Autodesk Inventor part; units mm, degrees
ref_plane "YZ Plane" through (0, 0, 0) normal (1, 0, 0) x (0, 1, 0)
ref_plane "XZ Plane" through (0, 0, 0) normal (0, 1, 0) x (-1, 0, 0)
ref_plane "XY Plane" through (0, 0, 0) normal (0, 0, 1) x (1, 0, 0)
sketch "Sketch1" plane through (0, 0, 0) normal (0, 0, 1) x (1, 0, 0)
  line L0 (-15.1032, 11.1381) -> (-28.4636, 11.1381)
  line L1 (-28.4636, 11.1381) -> (-28.4636, 26.8861)
  line L2 (-28.4636, 26.8861) -> (-15.1032, 26.8861)
  line L3 (-15.1032, 26.8861) -> (-15.1032, 11.1381)
  dimension "d0" = 13.3604
  dimension "d1" = 15.748
extrude "Extrusion1" add sketch "Sketch1" along normal blind 13.3096
sketch "Sketch2" plane through (0, 0, 13.3096) normal (0, 0, 1) x (1, 0, 0)
  line L0 (-28.4636, 11.1381) -> (-28.4636, 26.8861)
  line L1 (-15.1032, 11.1381) -> (-28.4636, 11.1381)
  line L2 (-15.1032, 26.8861) -> (-15.1032, 11.1381)
  line L3 (-28.4636, 26.8861) -> (-15.1032, 26.8861)
  line L4 (-23.79, 26.3273) -> (-19.7768, 26.3273)
  line L5 (-19.7768, 26.3273) -> (-19.7768, 24.0413)
  line L6 (-19.7768, 24.0413) -> (-23.79, 24.0413)
  line L7 (-23.79, 24.0413) -> (-23.79, 26.3273)
  line L8 (-25.06, 24.0413) -> (-18.5068, 24.0413)
  line L9 (-18.5068, 24.0413) -> (-18.5068, 22.8221)
  line L10 (-18.5068, 22.8221) -> (-25.06, 22.8221)
  line L11 (-25.06, 22.8221) -> (-25.06, 24.0413)
  line L12 (-16.5764, 22.8221) -> (-26.9904, 22.8221)
  line L13 (-26.9904, 22.8221) -> (-26.9904, 15.1259)
  line L14 (-26.9904, 15.1259) -> (-16.5764, 15.1259)
  line L15 (-16.5764, 15.1259) -> (-16.5764, 22.8221)
  line L16 (-25.06, 15.1259) -> (-18.5068, 15.1259)
  line L17 (-18.5068, 15.1259) -> (-18.5068, 14.0337)
  line L18 (-18.5068, 14.0337) -> (-25.06, 14.0337)
  line L19 (-25.06, 14.0337) -> (-25.06, 15.1259)
  dimension "d4" = 0.5588
  dimension "d5" = 4.6736
  dimension "d6" = 4.6736
  dimension "d7" = 2.286
  dimension "d9" = 1.27
  dimension "d10" = 1.27
  dimension "d11" = 1.2192
  dimension "d13" = 6.5532
  dimension "d14" = 1.9304
  dimension "d15" = 1.9304
  dimension "d16" = 10.414
  dimension "d17" = 7.6962
  dimension "d18" = 1.9304
  dimension "d19" = 1.9304
  dimension "d20" = 1.0922
  dimension "d21" = 2.8956
extrude "Extrusion2" cut sketch "Sketch2" against normal blind 14.1478 contours L4 L5 L6 L7 | L6 L8 L9 L10 L11 | L10 L12 L15 L14 L13 | L14 L17 L18 L19
sketch "Sketch3" plane through (0, 0, 0) normal (0, 0, -1) x (-1, 0, 0)
  line L0 (15.1032, 11.1381) -> (28.4636, 11.1381)
  line L1 (28.4636, 11.1381) -> (28.4636, 26.8861)
  line L2 (28.4636, 26.8861) -> (15.1032, 26.8861)
  line L3 (15.1032, 26.8861) -> (15.1032, 11.1381)
extrude "Extrusion3" add sketch "Sketch3" against normal blind 0.127
sketch "Sketch4" plane through (0, 0, 0.127) normal (0, 0, 1) x (1, 0, 0)
  line L0 (-25.06, 14.0337) -> (-25.06, 15.1259)
  line L1 (-18.5068, 14.0337) -> (-25.06, 14.0337)
  line L2 (-18.5068, 15.1259) -> (-18.5068, 14.0337)
  line L3 (-22.8629, 14.0337) -> (-22.6089, 14.0337)
  line L4 (-22.6089, 14.0337) -> (-22.6089, 16.4931)
  line L5 (-22.6089, 16.4931) -> (-22.8629, 16.4931)
  line L6 (-22.8629, 16.4931) -> (-22.8629, 14.0337)
  line L7 (-22.2279, 14.0337) -> (-21.9739, 14.0337)
  line L8 (-21.9739, 14.0337) -> (-21.9739, 16.4931)
  line L9 (-21.9739, 16.4931) -> (-22.2279, 16.4931)
  line L10 (-22.2279, 16.4931) -> (-22.2279, 14.0337)
  line L11 (-21.5929, 14.0337) -> (-21.3389, 14.0337)
  line L12 (-21.3389, 14.0337) -> (-21.3389, 16.4931)
  line L13 (-21.3389, 16.4931) -> (-21.5929, 16.4931)
  line L14 (-21.5929, 16.4931) -> (-21.5929, 14.0337)
  line L15 (-20.9579, 14.0337) -> (-20.7039, 14.0337)
  line L16 (-20.7039, 14.0337) -> (-20.7039, 16.4931)
  line L17 (-20.7039, 16.4931) -> (-20.9579, 16.4931)
  line L18 (-20.9579, 16.4931) -> (-20.9579, 14.0337)
  dimension "d26" = 0.254
  dimension "d27" = 0.254
  dimension "d28" = 0.254
  dimension "d29" = 0.254
  dimension "d30" = 0.381
  dimension "d31" = 0.381
  dimension "d32" = 0.381
  dimension "d33" = 2.1971
  dimension "d34" = 2.1971
extrude "Extrusion4" add sketch "Sketch4" along normal blind 6.4516
sketch "Sketch5" plane through (-22.8629, 14.0337, 0.127) normal (-1, 0, 0) x (0, 0, 1)
  line L0 (6.4516, 0) -> (6.4516, 2.4594)
  line L1 (0, 2.4594) -> (6.4516, 2.4594)
  line L2 (6.4516, 0) -> (0.1115, 2.4594)
extrude "Extrusion5" cut sketch "Sketch5" against normal blind 3.81
fillet "Fillet1" radius 0.127 8 edges at (-22.8629, 15.2634, 3.4085) (-22.6089, 15.2634, 3.4085) (-21.9739, 15.2634, 3.4085) (-22.2279, 15.2634, 3.4085) (-21.5929, 15.2634, 3.4085) (-21.3389, 15.2634, 3.4085) (-20.9579, 15.2634, 3.4085) (-20.7039, 15.2634, 3.4085)
sketch "Sketch6" plane through (0, 0, 0.127) normal (0, 0, 1) x (1, 0, 0)
  line L0 (-22.6089, 16.4001) -> (-22.6089, 14.0337)
  line L1 (-21.9739, 16.4001) -> (-21.9739, 14.0337)
  line L2 (-21.3389, 16.4001) -> (-21.3389, 14.0337)
  line L3 (-20.7039, 16.4001) -> (-20.7039, 14.0337)
  line L4 (-18.5068, 14.0337) -> (-20.7039, 14.0337)
  line L5 (-22.8629, 14.0337) -> (-25.06, 14.0337)
  line L6 (-22.8629, 14.0337) -> (-22.8629, 16.4001)
  line L7 (-25.0727, 14.0337) -> (-22.8629, 14.0337)
  line L8 (-22.8629, 14.0337) -> (-22.8629, 15.1259)
  line L9 (-22.8629, 15.1259) -> (-25.0727, 15.1259)
  line L10 (-25.0727, 15.1259) -> (-25.0727, 14.0337)
  line L11 (-22.6089, 15.1259) -> (-22.2279, 15.1259)
  line L12 (-22.2279, 15.1259) -> (-22.2279, 14.0337)
  line L13 (-22.2279, 14.0337) -> (-22.6089, 14.0337)
  line L14 (-22.6089, 14.0337) -> (-22.6089, 15.1259)
  line L15 (-21.9739, 15.1259) -> (-21.5929, 15.1259)
  line L16 (-21.5929, 15.1259) -> (-21.5929, 14.0337)
  line L17 (-21.5929, 14.0337) -> (-21.9739, 14.0337)
  line L18 (-21.9739, 14.0337) -> (-21.9739, 15.1259)
  line L19 (-21.3389, 15.1259) -> (-20.9579, 15.1259)
  line L20 (-20.9579, 15.1259) -> (-20.9579, 14.0337)
  line L21 (-20.9579, 14.0337) -> (-21.3389, 14.0337)
  line L22 (-21.3389, 14.0337) -> (-21.3389, 15.1259)
  line L23 (-20.7039, 15.1259) -> (-18.4941, 15.1259)
  line L24 (-18.4941, 15.1259) -> (-18.4941, 14.0337)
  line L25 (-18.4941, 14.0337) -> (-20.7039, 14.0337)
  line L26 (-20.7039, 14.0337) -> (-20.7039, 15.1259)
  line L27 (-22.8629, 14.0337) -> (-25.0727, 14.0337)
  line L28 (-25.0727, 14.0337) -> (-25.0727, 15.1259)
  line L29 (-25.0727, 15.1259) -> (-22.8629, 15.1259)
  line L30 (-22.8629, 15.1259) -> (-22.8629, 14.0337)
  line L31 (-20.7039, 15.1259) -> (-18.4941, 15.1259)
  line L32 (-18.4941, 15.1259) -> (-18.4941, 14.0337)
  line L33 (-18.4941, 14.0337) -> (-20.7039, 14.0337)
  line L34 (-20.7039, 14.0337) -> (-20.7039, 15.1259)
  point P0 (-25.06, 15.1259)
  dimension "d40" = 1.0922
  dimension "d41" = 1.0922
  dimension "d42" = 0
  dimension "d43" = 0
  dimension "d44" = 0
  dimension "d45" = 0
  dimension "d46" = 2.2098
  dimension "d47" = 2.2098
extrude "Extrusion6" add sketch "Sketch6" along normal blind 6.4516
sketch "Sketch7" plane through (0, 0, 0.127) normal (0, 0, 1) x (1, 0, 0)
  line L0 (-22.8629, 15.1259) -> (-22.6089, 15.1259)
  line L1 (-22.6089, 15.1259) -> (-22.6089, 22.5284)
  line L2 (-22.6089, 22.5284) -> (-22.8629, 22.5284)
  line L3 (-22.8629, 22.5284) -> (-22.8629, 15.1259)
  line L4 (-22.2279, 15.1259) -> (-21.9739, 15.1259)
  line L5 (-21.9739, 15.1259) -> (-21.9739, 22.5284)
  line L6 (-21.9739, 22.5284) -> (-22.2279, 22.5284)
  line L7 (-22.2279, 22.5284) -> (-22.2279, 15.1259)
  line L8 (-21.5929, 15.1259) -> (-21.3389, 15.1259)
  line L9 (-21.3389, 15.1259) -> (-21.3389, 22.5284)
  line L10 (-21.3389, 22.5284) -> (-21.5929, 22.5284)
  line L11 (-21.5929, 22.5284) -> (-21.5929, 15.1259)
  line L12 (-20.9579, 15.1259) -> (-20.7039, 15.1259)
  line L13 (-20.7039, 15.1259) -> (-20.7039, 22.5284)
  line L14 (-20.7039, 22.5284) -> (-20.9579, 22.5284)
  line L15 (-20.9579, 22.5284) -> (-20.9579, 15.1259)
  line L16 (-22.9407, 16.4931) -> (-20.3193, 16.4931)
  line L17 (-20.7381, 16.4931) -> (-20.9579, 16.4931)
  line L18 (-20.9579, 16.4931) -> (-20.9579, 22.5284)
  line L19 (-20.9579, 22.5284) -> (-20.7381, 22.5284)
  line L20 (-21.5929, 22.5284) -> (-21.3731, 22.5284)
  line L21 (-21.3731, 16.4931) -> (-21.5929, 16.4931)
  line L22 (-21.5929, 16.4931) -> (-21.5929, 22.5284)
  line L23 (-20.7039, 16.4931) -> (-20.9579, 16.4931)
  line L24 (-20.9579, 16.4931) -> (-20.9579, 22.5284)
  line L25 (-20.9579, 22.5284) -> (-20.7039, 22.5284)
  line L26 (-20.7039, 22.5284) -> (-20.7039, 16.4931)
  line L27 (-21.5929, 22.5284) -> (-21.3389, 22.5284)
  line L28 (-21.3389, 22.5284) -> (-21.3389, 16.4931)
  line L29 (-21.3389, 16.4931) -> (-21.5929, 16.4931)
  line L30 (-21.5929, 16.4931) -> (-21.5929, 22.5284)
  line L31 (-21.9739, 16.4931) -> (-22.2279, 16.4931)
  line L32 (-22.2279, 16.4931) -> (-22.2279, 22.5284)
  line L33 (-22.2279, 22.5284) -> (-21.9739, 22.5284)
  line L34 (-21.9739, 22.5284) -> (-21.9739, 16.4931)
  line L35 (-22.8629, 22.5284) -> (-22.6089, 22.5284)
  line L36 (-22.6089, 22.5284) -> (-22.6089, 16.4931)
  line L37 (-22.6089, 16.4931) -> (-22.8629, 16.4931)
  line L38 (-22.8629, 16.4931) -> (-22.8629, 22.5284)
extrude "Extrusion7" cut sketch "Sketch7" against normal blind 127 contours L15 L14 L13 L16 | L11 L10 L9 L16 | L7 L6 L5 L16 | L3 L2 L1 L16
equation "\"d6\" = d5"
equation "\"d10\" = d9"
equation "\"d15\" = d14"
equation "\"d27\" = d26"
equation "\"d28\" = d27"
equation "\"d29\" = d28"
equation "\"d31\" = d30"
equation "\"d32\" = d31"
equation "\"d40\" = d41"
equation "\"d47\" = d46"
properties part number "2009_CTS_EatherNetPort"
Geometry: final body of the model. Coordinates: model frame, mm. Coordinates: 2 decimals unless noted, no trailing zeros. Order: outer loops, then holes, each group sorted by start corner. A loop starts at its lowest first (then second) coordinate and runs counter-clockwise, first axis right, second up. Notation, with made-up numbers: M 43,75 L 83,75 A26 cw 83,97 Z; hole C 73.25,-4 d2. An arc over 180 degrees is marked long. Answer in a Markdown table with one row per item. Add a question column.
Q1. Line query: L1, parallel to X at y = 21, z = 7.25; L2, parallel to Y at x = -20.5, z = 8.75; L3, parallel to Y at x = -17, z = 3.5. Output: solid intervals per line, ascending.
Q2. Section query A-A on z = 11.5. Return the cut outline in (x, y).
Q3. Mould query, pull axis Z, two halves, no side actions, for faces 1 (the flat face through (-23.79, 25, 7)), 2 (the flat face through (-24, 14.6, 6.579)). Classes: released by +Z, released by -Z, zero draft, split by the parting line, or undercut.
Q4. Section query D-D on y = 23.75. Return the cut outline in (x, z).
Q5. Section query C-C on x = -17.75. Return the cut outline in (y, z), and give its area (3 significant figures).
Q6. Section query B-B on y = 19.25. Return the cut outline in (x, z), and give its area (3 significant figures).
Q7. Contact query for a flat-ended pin moving along its axis: P1, Ø4, axis at x = -25.5, y = 17, coming from the -Z side. Output: stop coordinate, or through.
Completed:
| question | item | result |
|---|---|---|
| 1 | L1 | x = -28.46 to -26.99, -16.58 to -15.1 |
| 1 | L2 | y = 11.14 to 14.03, 26.33 to 26.89 |
| 1 | L3 | y = 11.14 to 15.13, 22.82 to 26.89 |
| 2 | outline | M -28.46,11.14 L -15.1,11.14 L -15.1,26.89 L -28.46,26.89 Z; hole M -26.99,15.13 L -25.06,15.13 L -25.06,14.03 L -18.51,14.03 L -18.51,15.13 L -16.58,15.13 L -16.58,22.82 L -18.51,22.82 L -18.51,24.04 L -19.78,24.04 L -19.78,26.33 L -23.79,26.33 L -23.79,24.04 L -25.06,24.04 L -25.06,22.82 L -26.99,22.82 Z |
| 3 | face 1 | zero draft |
| 3 | face 2 | released by +Z |
| 4 | outline | M -28.46,0 L -15.1,0 L -15.1,13.31 L -18.51,13.31 L -18.51,0.13 L -25.06,0.13 L -25.06,13.31 L -28.46,13.31 Z |
| 5 | outline | M 11.14,0 L 26.89,0 L 26.89,13.31 L 22.82,13.31 L 22.82,0.13 L 15.13,0.13 L 15.13,13.31 L 11.14,13.31 Z |
| 5 | area | 108 mm2 |
| 6 | outline | M -28.46,0 L -22.86,0 L -22.86,0.13 L -26.99,0.13 L -26.99,13.31 L -28.46,13.31 Z; M -22.61,0 L -22.23,0 L -22.23,0.13 L -22.61,0.13 Z; M -21.97,0 L -21.59,0 L -21.59,0.13 L -21.97,0.13 Z; M -21.34,0 L -20.96,0 L -20.96,0.13 L -21.34,0.13 Z; M -20.7,0 L -15.1,0 L -15.1,13.31 L -16.58,13.31 L -16.58,0.13 L -20.7,0.13 Z |
| 6 | area | 40.4 mm2 |
| 7 | P1 | stops at z = 0 |
